Input: part model. Units: mm. Frame: model coordinates. A direction names the side the tool comes from. Coordinates: 2 decimals unless noted, no trailing zeros. Loops run counter-clockwise (first coordinate to the right, second up) from the corner with the lowest first, then second, coordinate; pieces in that order, holes last. Notation, with made-up numbers: (-20.5, -31.75) -> (-8.5, -31.75) arc R32 cw to (-8.5, 1.25) -> close; hole circle Ø10 at (15, 89.25). An arc over 180 degrees is marked (long way). Answer as a JSON object with one key per item and string values.
Autodesk Inventor part; units mm, degrees
ref_plane "Plano de trabajo1" through (-2.2861, 0, 1.3081) normal (-0.5, 0, -0.8661) x (-0.8661, 0, 0.5)
ref_plane "Plano de trabajo2" through (4.5, 0, -2.5981) normal (0.5, 0, 0.866) x (0, 1, 0)
ref_plane "YZ Plane" through (0, 0, 0) normal (1, 0, 0) x (0, 1, 0)
sketch "Boceto1" plane through (0, 0, 0) normal (0, 1, 0) x (-1, 0, 0)
  circle A0 centre (0, 0) radius 4.5
  dimension "d0" = 9
extrude "Extrusión1" add sketch "Boceto1" along normal blind 64.47
fillet "Empalme1" radius 4.5 1 edges at (4.5, 64.47, 0)
sketch "Boceto2" plane through (0, 0, 0) normal (0, -1, 0) x (1, 0, 0)
  circle A0 centre (0, 0) radius 4.5
  circle A1 centre (0, 0) radius 4.5
  line L0 (3.8723, -2.2357) -> (3.8971, -2.25)
  line L1 (0, 0) -> (5.1962, 0) construction
  line L2 (4.5, -2.5981) -> (4.5, 2.5981)
  line L3 (0, 0) -> (5.1962, 0) construction
  line L4 (4.5, 2.5981) -> (0, 5.1958)
  line L5 (0, 5.1958) -> (-4.5, 2.5981)
  line L6 (-4.5, 2.5981) -> (-4.5409, -2.5978)
  line L7 (-4.5409, -2.5978) -> (-0.0409, -5.1955)
  line L8 (-0.0409, -5.1955) -> (4.5, -2.5981)
  dimension "d9" = 30
  dimension "d11" = 5.196
  dimension "d12" = 5.196
  dimension "d13" = 5.196
  dimension "d14" = 5.196
extrude "Extrusión2" add sketch "Boceto2" against normal blind 16.1175 contours A0 L8 | A0 L2 L8 | A0 L4 L2 | A0 L5 L4 | L8 L7 L6 L5 A0 picked at (-2.0247, -0.1583)
ref_plane "Plano de trabajo1" through (-2.2861, 0, 1.3081) normal (-0.5, 0, -0.8661) x (-0.8661, 0, 0.5)
ref_plane "Plano de trabajo2" through (4.5, 0, -2.5981) normal (0.5, 0, 0.866) x (0, 1, 0)
properties part number "antena"
1. Pin query (flat end, axial travel): P1, Ø5, axis at x = 3.5, z = 0.5, coming from the +Y side; P2, Ø1.4, axis at x = 0, z = 4.5, coming from the +Y side; P3, Ø2, axis at x = 3.5, z = -2.5, coming from the +Y side. Return the tip coordinate at first contact, or that it passes through.
Reply:
{"P1": "stops at y = 64.35", "P2": "stops at y = 62.38", "P3": "stops at y = 63.03"}
2. Section query B-B (x = 3.5). Return loops of the section in (y, z).
Reply:
{"outline": "(0, -3.17) -> (16.12, -3.17) -> (16.12, -2.83) -> (59.97, -2.83) arc R2.83 ccw to (59.97, 2.83) -> (16.12, 2.83) -> (16.12, 3.18) -> (0, 3.18) -> close"}
3. Line query: line 1 along X through (y, z) = (11.5, 1.5); line 2 along Y through (x, z) = (0, 0.5); line 3 along X through (y, z) = (37.5, -4). Output: solid intervals per line, ascending.
Reply:
{"line 1": "x = -4.51 to 4.5", "line 2": "y = 0 to 64.44", "line 3": "x = -2.06 to 2.06"}
4. Section query C-C (y = 43). Return loops of the section in (x, z).
Reply:
{"outline": "circle Ø9 at (0, 0)"}
5. Section query A-A (y = 5.5). Return loops of the section in (x, z).
Reply:
{"outline": "(-4.54, -2.6) -> (-0.04, -5.2) -> (1.96, -4.05) arc R4.5 ccw to (2.5, -3.74) -> (4.5, -2.6) -> (4.5, 2.6) -> (0, 5.2) -> (-4.5, 2.6) -> close"}
6. Access query for faces 1 (the face through (0.59, 36.23, -4.46)), 2 (the face through (4.1, 16.118, -2.3)), 3 (the face through (4, 16.118, 2.4)), 4 (the face through (-2.32, 7.95, -3.88)). Directions: +Z, -Z, +X, -X, +Y, -Y. A direction counts if a zero-diameter tool reaches every point of the face in a straight line with its end or side. Return the directions, or none.
Reply:
{"face 1": "+Y", "face 2": "-Z, +X, +Y", "face 3": "+Z, +X, +Y", "face 4": "-Z, -X, +Y, -Y"}
